Model file for the job. Use its own axes, mm. A direction names the side the tool comes from. Coordinates: 2 decimals unless noted, no trailing zeros. Loops run counter-clockwise (first coordinate to the right, second up) from the corner with the lowest first, then second, coordinate; pieces in that order, holes last. Notation, with made-up numbers: (51, -38) - (72, -38) arc R23 ccw to (72, 0) - close; hole circle Ø10 at (52.25, 26). An arc over 180 degrees is marked (long way). Write each question's results on one line, items separated by ' | '. Start each with the question number.
```python
from build123d import *

# Parameters (mm, degrees)
SKETCH1_R                = 20
BOSS_EXTRUDE2_DEPTH      = 56
SKETCH1_4_R              = 1.5
BOSS_EXTRUDE3_DEPTH      = 2
SKETCH1_5_R              = 9
SKETCH1_5_R_2            = 2.5
BOSS_EXTRUDE4_DEPTH      = 4
SKETCH1_7_R              = 2.5
BOSS_EXTRUDE6_DEPTH      = 65
BOSS_EXTRUDE6_DEPTH_BACK = 17
SKETCH8_R                = 24
SKETCH8_R_2              = 2.5
BOSS_EXTRUDE9_DEPTH      = 2
SKETCH9_R                = 2.5
BOSS_EXTRUDE11_DEPTH     = 10


with BuildPart() as part:
    # Sketch1 → Boss-Extrude2 (new body)
    with BuildSketch(Plane.XY):
        with Locations((-44.212108768, 22.898771409)):
            Circle(SKETCH1_R)
    extrude(amount=BOSS_EXTRUDE2_DEPTH)

    # Sketch1_4 → Boss-Extrude3 (add)
    with BuildSketch(Plane.XY):
        with BuildLine():
            Line((-71.211826981, 24.398484848), (-71.211826981, 21.399057969))
            Line((-71.211826981, 21.399057969), (-59.405868846, 9.893016732))
            ThreePointArc((-59.405868846, 9.893016732), (-64.212108768, 22.898771409), (-59.405868846, 35.904526085))
            Line((-59.405868846, 35.904526085), (-71.211826981, 24.398484848))
        make_face()
        with Locations((-67.212108768, 22.898771409)):
            Circle(SKETCH1_4_R, mode=Mode.SUBTRACT)
        with BuildLine():
            ThreePointArc((-29.018348691, 35.904526085), (-24.212108768, 22.898771409), (-29.018348691, 9.893016732))
            Line((-29.018348691, 9.893016732), (-17.212390555, 21.399057969))
            Line((-17.212390555, 21.399057969), (-17.212390555, 24.398484848))
            Line((-17.212390555, 24.398484848), (-29.018348691, 35.904526085))
        make_face()
        with Locations((-21.212108768, 22.898771409)):
            Circle(SKETCH1_4_R, mode=Mode.SUBTRACT)
    extrude(amount=BOSS_EXTRUDE3_DEPTH)

    # Sketch1_5 → Boss-Extrude4 (add)
    with BuildSketch(Plane.XY):
        with Locations((-44.212108768, 22.898771409)):
            Circle(SKETCH1_5_R)
        with Locations((-44.212108768, 22.898771409)):
            Circle(SKETCH1_5_R_2, mode=Mode.SUBTRACT)
    extrude(amount=-BOSS_EXTRUDE4_DEPTH)

    # Sketch1_7 → Boss-Extrude6 (add, two sides)
    with BuildSketch(Plane.XY) as boss_extrude6_sk:
        with Locations((-44.212108768, 22.898771409)):
            Circle(SKETCH1_7_R)
    extrude(amount=BOSS_EXTRUDE6_DEPTH)
    extrude(boss_extrude6_sk.sketch, amount=-BOSS_EXTRUDE6_DEPTH_BACK)

    # Sketch8 → Boss-Extrude9 (add)
    with BuildSketch(Plane.XY.offset(65)):
        with Locations((-44.212108768, 22.898771409)):
            Circle(SKETCH8_R)
        with Locations((-44.212108768, 22.898771409)):
            Circle(SKETCH8_R_2, mode=Mode.SUBTRACT)
    extrude(amount=-BOSS_EXTRUDE9_DEPTH)

    # Sketch9 → Boss-Extrude11 (add)
    with BuildSketch(Plane.XY.offset(65)):
        with Locations((-44.212108768, 22.898771409)):
            Circle(SKETCH9_R)
    extrude(amount=BOSS_EXTRUDE11_DEPTH)


solid = part.part
```
Q1. Drill centre lines: L1, parallel to Z at x = -36, y = 15.5; L2, parallel to Z at x = -49, y = 27; L3, parallel to Z at x = -24, y = 35. Where is each one in solid material? Low to high. Write a range as from..to.
Q2. Mould opens along Z. For faces 1 (the flat face through (-65, 23, 2)), 2 (the cylindrical face through (-41.903, 21.941, -10.409)), 3 (the flat face through (-44.6, 32.1, 0)) say: +Z half, -Z half, draft (parallel to the pull), parting line (faces both ways), or undercut.
Q3. Cut at D-D (x = -36.5). List the corners of the cut face in (y, z).
Q4. Which spindle directions (+Z, -Z, +X, -X, +Y, -Y) get a long thin tool onto all of the face, cutting with end or side? Do faces 4 (the cylindrical face through (-35.628, 25.602, -1.972)), 5 (the cylindrical face through (-41.903, 21.941, 69.93)), 6 (the flat face through (-23.03, 30.07, 0.99)), 7 (the flat face through (-65.391, 15.727, 0.986)). Say none if no direction does.
Q5. Cut at C-C (z = 1). List the corners of the cut face in (x, y).
Q6. Cut at A-A (y = 27.5). List the corners of the cut face in (x, z), and give its area (3 significant figures).
Q7. Pin check, flat tips, straight feed: pin 1 (12 mm diameter, centred on x = -65, z = 41, fed in from -Y); pin 2 (4 mm diameter, centred on y = 32, z = -4.5, fed in from +X); pin 3 (10 mm diameter, centred on y = 22.5, z = 9, fed in from +X). Stop position of each tip, or through.
Q8. Cut at B-B (x = -57.5). List the corners of the cut face in (y, z).
Check result:
1) L1: 0..56, 63..65 | L2: -4..56, 63..65 | L3: 63..65
2) face 1: undercut | face 2: draft | face 3: -Z half
3) outline: (0.17, 63) - (45.63, 63) - (45.63, 65) - (0.17, 65) - close; (4.45, 0) - (18.26, 0) - (18.26, -4) - (27.54, -4) - (27.54, 0) - (41.35, 0) - (41.35, 56) - (4.45, 56) - close
4) face 4: -Z | face 5: +Z | face 6: -Z, +X, +Y | face 7: -Z, -X, -Y
5) outline: (-71.21, 21.4) - (-59.41, 9.89) arc R20 ccw to (-29.02, 9.89) - (-17.21, 21.4) - (-17.21, 24.4) - (-29.02, 35.9) arc R20 ccw to (-59.41, 35.9) - (-71.21, 24.4) - close; hole circle Ø3 at (-67.21, 22.9); hole circle Ø3 at (-21.21, 22.9)
6) outline: (-68.03, 0) - (-51.95, 0) - (-51.95, -4) - (-36.48, -4) - (-36.48, 0) - (-20.39, 0) - (-20.39, 2) - (-24.75, 2) - (-24.75, 56) - (-63.68, 56) - (-63.68, 2) - (-68.03, 2) - close; (-67.77, 63) - (-20.66, 63) - (-20.66, 65) - (-67.77, 65) - close | area: 2,350 mm²
7) pin 1: y = 9.43 | pin 2: x = -38.77 | pin 3: x = -24.21
8) outline: (2.91, 63) - (42.88, 63) - (42.88, 65) - (2.91, 65) - close; (7.95, 0) - (37.85, 0) - (37.85, 56) - (7.95, 56) - close
